```python
from build123d import *

# Parameters (mm, degrees)
SKETCH1_R               = 8.89
SKETCH1_R_2             = 4.572
BOSS_EXTRUDE1_DEPTH     = 6.35
CUT_EXTRUDE1_REACH      = 16.085
CUT_EXTRUDE1_END_RADIUS = 8.89
SKETCH2_R               = 0.889
CUT_EXTRUDE2_REACH      = 16.085
CUT_EXTRUDE2_END_RADIUS = 8.89
SKETCH3_R               = 0.889


with BuildPart() as part:
    # Sketch1 → Boss-Extrude1 (new body)
    with BuildSketch(Plane(origin=(0, 0, 0), x_dir=(1, 0, 0), z_dir=(0, 1, 0))):
        with Locations(Location((0, 0, 0), (0, 0, 270))):
            Circle(SKETCH1_R)
        with Locations(Location((0, 0, 0), (0, 0, 270))):
            Circle(SKETCH1_R_2, mode=Mode.SUBTRACT)
    extrude(amount=BOSS_EXTRUDE1_DEPTH)

    # Cut-Extrude1: up to this cylinder (the profile starts inside it)
    cut_extrude1_end = Plane(origin=(0, 3.175, 0), z_dir=(0, -1, 0)) * Cylinder(CUT_EXTRUDE1_END_RADIUS, 50.95, mode=Mode.PRIVATE)
    # Sketch2 → Cut-Extrude1 (cut, up to the surface)
    with BuildSketch(Plane(origin=(0, 0, 0), x_dir=(0, 0, -1), z_dir=(1, 0, 0)), mode=Mode.PRIVATE) as cut_extrude1_sk1:
        with Locations(Location((0, 3.175, 0), (0, 0, 180))):
            Circle(SKETCH2_R)
    cut_extrude1_tool1 = extrude(cut_extrude1_sk1.sketch, amount=CUT_EXTRUDE1_REACH, mode=Mode.PRIVATE) & cut_extrude1_end
    add(cut_extrude1_tool1.solids().sort_by_distance((0, 3.175, 0))[0], mode=Mode.SUBTRACT)

    # Cut-Extrude2: up to this cylinder (the profile starts inside it)
    cut_extrude2_end = Plane(origin=(0, 3.175, 0), z_dir=(0, -1, 0)) * Cylinder(CUT_EXTRUDE2_END_RADIUS, 50.95, mode=Mode.PRIVATE)
    # Sketch3 → Cut-Extrude2 (cut, up to the surface)
    with BuildSketch(Plane.XY, mode=Mode.PRIVATE) as cut_extrude2_sk1:
        with Locations(Location((0, 3.175, 0), (0, 0, 180))):
            Circle(SKETCH3_R)
    cut_extrude2_tool1 = extrude(cut_extrude2_sk1.sketch, amount=CUT_EXTRUDE2_REACH, mode=Mode.PRIVATE) & cut_extrude2_end
    add(cut_extrude2_tool1.solids().sort_by_distance((0, 3.175, 0))[0], mode=Mode.SUBTRACT)


solid = part.part
```
Part model, mm, in its own coordinate system. Give positions to 0.01 mm unless a question says otherwise; leave off trailing zeros. Write each loop counter-clockwise with the first axis right and the second up, starting at its lowest first coordinate (ties: lowest second). Pieces come first, ordered by that corner, then holes. Notation, with made-up numbers: (-2.5, -21.5) -> (14.5, -21.5) arc R20 cw to (14.5, 11.5) -> close; hole circle Ø1 at (19.25, -29). An arc over 180 degrees is marked (long way). Put each result on its own line as item: value. Start each with the question number.
Item 1: Cut at A-A (z = 0). List the corners of the cut face in (x, y), then the cut area to 3 significant figures.
Item 2: Pin check, flat tips, straight feed: pin 1 Ø1 at (y, z) = (4, -2.5) entering from -X; pin 2 Ø2 at (x, y) = (-4.5, 0.5) entering from -Z; pin 3 Ø3 at (x, y) = (3, 3) entering from +Z. Stop position of each tip, or through.
Item 3: Wall check: L1, parallel to X at y = 4.75, z = 0; L2, parallel to Y at x = 0, z = 6.4; L3, parallel to Z at x = -2.5, y = 4.5. Give the ranges that are in metal, low to high. Write a range as [from, to].
Item 4: Cut at C-C (y = 3.5). List the corners of the cut face in (x, z).
Item 5: Pull direction Y, two halves, no side cores. Call faces 1 (the face through (-4, 0, 4)), 2 (the face through (6.657, 4.043, -0.193)), 3 (the face through (0.193, 4.043, 6.657)), 4 (the face through (-4, 6.35, 4)): pulls with the +Y half, pulls with the -Y half, needs draft (parallel to the pull), parting line crosses it, or undercut.
Item 6: Cut at B-B (x = 0). List the corners of the cut face in (y, z), then the cut area to 3 significant figures.
Item 7: Cut at D-D (x = -4.25). List the corners of the cut face in (y, z), then the cut area to 3 significant figures.
Answer list:
1. outline: (-8.89, 0) -> (-4.57, 0) -> (-4.57, 6.35) -> (-8.89, 6.35) -> close; (4.57, 0) -> (8.89, 0) -> (8.89, 2.29) -> (4.57, 2.29) -> close; (4.57, 4.06) -> (8.89, 4.06) -> (8.89, 6.35) -> (4.57, 6.35) -> close
1. area: 47.2 mm2
2. pin 1: stops at x = -8.66
2. pin 2: stops at z = -8.17
2. pin 3: stops at z = 8.76
3. L1: x = [-8.89, -4.57], [4.57, 8.89]
3. L2: y = [0, 2.29], [4.06, 6.35]
3. L3: z = [-8.53, -3.83], [3.83, 8.53]
4. outline: (-0.83, 4.5) -> (-0.83, 8.85) arc R8.89 ccw (long way) to (8.85, -0.83) -> (4.5, -0.83) arc R4.57 cw (long way) to start; (0.83, 4.5) arc R4.57 cw to (4.5, 0.83) -> (8.85, 0.83) arc R8.89 ccw to (0.83, 8.85) -> close
5. face 1: pulls with the -Y half
5. face 2: undercut
5. face 3: undercut
5. face 4: pulls with the +Y half
6. outline: (0, -8.89) -> (6.35, -8.89) -> (6.35, -4.57) -> (0, -4.57) -> close; (0, 4.57) -> (2.29, 4.57) -> (2.29, 8.89) -> (0, 8.89) -> close; (4.06, 4.57) -> (6.35, 4.57) -> (6.35, 8.89) -> (4.06, 8.89) -> close
6. area: 47.2 mm2
7. outline: (0, -7.81) -> (6.35, -7.81) -> (6.35, -1.69) -> (0, -1.69) -> close; (0, 1.69) -> (6.35, 1.69) -> (6.35, 7.81) -> (0, 7.81) -> close
7. area: 77.8 mm2
